The drawing under review shows one solid part. Ordinate dimensions are in mm from its lowest x, y, z. A direction names the side the tool comes from. Round coordinates to 2 decimals unless told otherwise and drop trailing zeros. Order: outer loops, then holes, each group sorted by start corner. A loop starts at its lowest first (then second) coordinate and runs counter-clockwise, first axis right, second up.
1) To check wall thickness, follow L1, parallel to X at y = 70, z = 36 (1 decimal); L2, parallel to X at y = 43, z = 39.5 (1 decimal); L3, parallel to Z at x = 193.5, y = 28.5. State the ranges of each line that lie inside material, in increasing order.
2) Mouldability with a two-part tool opening along X and no side actions: class the marked faces 1, 2 and 3 as pulls with the +X half, pulls with the -X half, needs draft (parallel to the pull), parting line crosses it, or undercut.
3) Consider section D-D (x = 66.5). Give the boundary of the cut face in (y, z).
4) Clearance check with flat-ended pins moving along their axes: P1, Ø7.5, axis at x = 193.5, y = 54.5, coming from the -Z side; P2, Ø6.5, axis at x = 85.14, y = 26.46, coming from the -Z side; P3, Ø12, axis at x = 92.5, y = 56, coming from the +Z side; P4, Ø1.5, axis at x = 158.5, y = 15, coming from the -Z side (1 decimal). State where each tip first meets the part, or that it passes through.
5) Consider section B-B (y = 39). Give the boundary of the cut face in (x, z), then the cut area to 3 significant figures.
6) Consider section C-C (x = 154). Give the boundary of the cut face in (y, z), then the cut area to 3 significant figures.
7) Consider section A-A (z = 9). Give the boundary of the cut face in (x, y).
8) Machinability: for the marked faces 4, 5 and 6, which of the approach directions +Z, -Z, +X, -X, +Y, -Y give a long, thin tool a straight path to every point of the face, cutting with its end or side? Answer none if there is none.
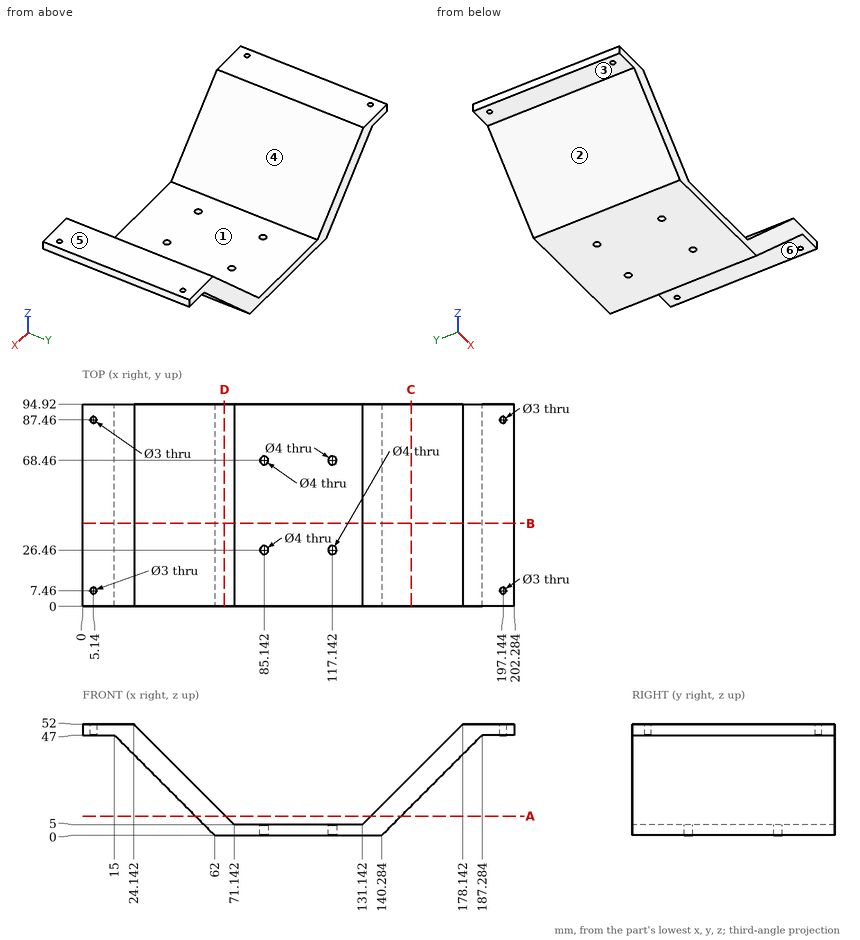
Answer below:
1. L1: x = 26 to 40.1, 162.1 to 176.3
1. L2: x = 22.5 to 36.6, 165.6 to 179.8
1. L3: z = 47 to 52
2. face 1: undercut
2. face 2: pulls with the -X half
2. face 3: needs draft
3. outline: (0, 0) - (94.92, 0) - (94.92, 9.64) - (0, 9.64) - close
4. P1: stops at z = 47
4. P2: stops at z = 0
4. P3: stops at z = 5
4. P4: stops at z = 17.5
5. outline: (0, 47) - (15, 47) - (62, 0) - (140.28, 0) - (187.28, 47) - (202.28, 47) - (202.28, 52) - (178.14, 52) - (131.14, 5) - (71.14, 5) - (24.14, 52) - (0, 52) - close
5. area: 1,870 mm2
6. outline: (0, 13.72) - (94.92, 13.72) - (94.92, 27.86) - (0, 27.86) - close
6. area: 1,340 mm2
7. outline: (53, 0) - (67.14, 0) - (67.14, 94.92) - (53, 94.92) - close; (135.14, 0) - (149.28, 0) - (149.28, 94.92) - (135.14, 94.92) - close
8. face 4: +Z, +Y, -Y
8. face 5: +Z, +X, -X, +Y, -Y
8. face 6: -Z, +X, +Y, -Y
